```python
from build123d import *

# Parameters (mm, degrees)
F0_R      = 10.795
F1_DEPTH  = 15.24
F1_FACE_R = 10.795
F2_DEPTH  = 5.08
F2_TAPER  = -20
F3_DEPTH  = 1.016
F5_DEPTH  = 6.0706


with BuildPart() as f1:
    # F0 (on Top) → F1 (new body)
    with BuildSketch(Plane.XY):
        Circle(F0_R)
    extrude(amount=F1_DEPTH)

    # F1_face (on face) → F2 (join)
    with BuildSketch(Plane.XY.offset(15.24)):
        Circle(F1_FACE_R)
    extrude(amount=F2_DEPTH, taper=F2_TAPER)

    # F3 (add): a face of the model
    f3_faces = [f1.faces().sort_by_distance(p)[0] for p in [
        (0, 0, 20.32),
    ]]
    extrude(f3_faces, amount=F3_DEPTH)

    # F4 (on face) → F5 (cut)
    with BuildSketch(Plane.XY.offset(21.336)):
        with BuildLine():
            Line((0.635, 7.1958522628), (-0.635, 7.1958522628))
            Line((-0.635, 7.1958522628), (-0.635, 1.0998522628))
            ThreePointArc((-0.635, 1.0998522628), (-0.8980256121, 0.8980256121), (-1.0998522628, 0.635))
            Line((-1.0998522628, 0.635), (-7.1958522628, 0.635))
            Line((-7.1958522628, 0.635), (-7.1958522628, -0.635))
            Line((-7.1958522628, -0.635), (-1.0998522628, -0.635))
            ThreePointArc((-1.0998522628, -0.635), (-0.8980256121, -0.8980256121), (-0.635, -1.0998522628))
            Line((-0.635, -1.0998522628), (-0.635, -7.1958522628))
            Line((-0.635, -7.1958522628), (0.635, -7.1958522628))
            Line((0.635, -7.1958522628), (0.635, -1.0998522628))
            ThreePointArc((0.635, -1.0998522628), (0.8980256121, -0.8980256121), (1.0998522628, -0.635))
            Line((1.0998522628, -0.635), (7.1958522628, -0.635))
            Line((7.1958522628, -0.635), (7.1958522628, 0.635))
            Line((7.1958522628, 0.635), (1.0998522628, 0.635))
            ThreePointArc((1.0998522628, 0.635), (0.8980256121, 0.8980256121), (0.635, 1.0998522628))
            Line((0.635, 1.0998522628), (0.635, 7.1958522628))
        make_face()
    extrude(amount=-F5_DEPTH, mode=Mode.SUBTRACT)

    # F6 (on Front) → F7 (revolve, cut)
    with BuildSketch(Plane.XZ):
        with BuildLine():
            ThreePointArc((0, 201.9231468439), (-90.8144451678, 111.1087016761), (0, 20.2942565084))
            Line((0, 20.2942565084), (0, 201.9231468439))
        make_face()
    revolve(axis=Axis((0, 0, 111.1087016761), (0, 0, 1)), mode=Mode.SUBTRACT)


solid = f1.part
```
Build history of the part. All positions in model axes, mm. A direction names the side the tool comes from. Round coordinates to 2 decimals unless told otherwise and drop trailing zeros. Write each loop counter-clockwise with the first axis right and the second up, starting at its lowest first coordinate (ties: lowest second). Pieces come first, ordered by that corner, then holes. Notation, with made-up numbers: (69.5, 79.25) -> (111.5, 79.25) arc R21 cw to (111.5, 90.25) -> close; hole circle Ø11 at (68, -23). An arc over 180 degrees is marked (long way). Put each result on its own line as item: value.
Item 1: Tool access for faces 4 (the face through (-10.034, 7.694, 20.743)), 5 (the face through (-7.956, 7.296, 7.513)), 6 (the face through (-4, 0.635, 18)): list every direction of +Z, -Z, +X, -X, +Y, -Y with a clear straight run to the whole face (end or side of a thin tool).
Here are the results:
face 4: +Z, -Z
face 5: -Z
face 6: +Z
Item 2: Slice it at A-A, the plane x = 0. Give the cut face in (y, z) (3 decimals), plus the area to 3 significant figures.
Here are the results:
outline: (-12.644, 20.32) -> (-10.795, 15.24) -> (-10.795, 0) -> (10.795, 0) -> (10.795, 15.24) -> (12.644, 20.32) -> (12.644, 21.179) arc R90.814 cw to (7.196, 20.58) -> (7.196, 15.265) -> (-7.196, 15.265) -> (-7.196, 20.58) arc R90.814 cw to (-12.644, 21.179) -> close
area: 381 mm^2
Item 3: Wall check: probe 1 along Z at (x, y) = (1.75, 1.5); probe 2 along Z at (x, y) = (0.75, 0.5); probe 3 along X at (y, z) = (-3.5, 16.25) (3 decimals). Give the ranges that are in metal, low to high. Write a range as from..to.
Here are the results:
probe 1: z = 0..20.32
probe 2: z = 0..15.27
probe 3: x = -10.6..-0.635, 0.635..10.6
Item 4: Two-plate mould, pull along Y, no slides. Class faces 1 (the face through (0, 0, 0)), 2 (the face through (10.407, 3.277, 15.558)), 3 (the face through (-0.635, -4, 18)): pulls with the +Y half, pulls with the -Y half, needs draft (parallel to the pull), parting line crosses it, or undercut.
Here are the results:
face 1: needs draft
face 2: parting line crosses it
face 3: undercut
Item 5: Slice it at C-C, the plane z = 5. Give the cut face in (x, y) (3 decimals).
Here are the results:
outline: circle Ø21.59 at (0, 0)
Item 6: Flat gauge pins, fed straight in: P1, Ø8, axis at x = -4, z = 13, coming from the +Y side; P2, Ø1.6, axis at y = 4, z = 16.5, coming from the -X side; P3, Ø2.5, axis at y = -3.5, z = 18.5, coming from the -X side. Where does each tip first touch, or does it go through?
Here are the results:
P1: stops at y = 11.06
P2: stops at x = -10.93
P3: stops at x = -12.04
Item 7: Slice it at B-B, the plane z = 18.25. Give the cut face in (x, y) (3 decimals).
Here are the results:
outline: circle Ø23.781 at (0, 0); hole (-7.196, -0.635) -> (-1.1, -0.635) arc R1.27 ccw to (-0.635, -1.1) -> (-0.635, -7.196) -> (0.635, -7.196) -> (0.635, -1.1) arc R1.27 ccw to (1.1, -0.635) -> (7.196, -0.635) -> (7.196, 0.635) -> (1.1, 0.635) arc R1.27 ccw to (0.635, 1.1) -> (0.635, 7.196) -> (-0.635, 7.196) -> (-0.635, 1.1) arc R1.27 ccw to (-1.1, 0.635) -> (-7.196, 0.635) -> close
